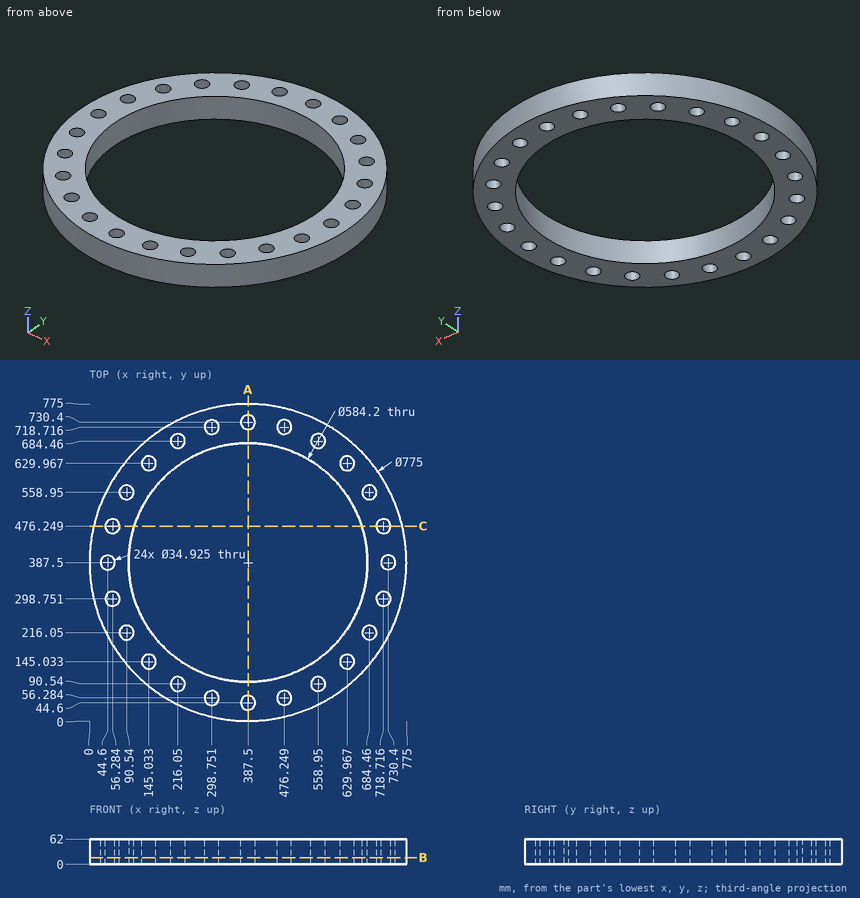
Check sheet for the drawn part. Datum: minimum x, y, z corner. Units: mm. Round coordinates to 2 decimals unless told otherwise and drop trailing zeros. Order: outer loops, then holes, each group sorted by start corner. A loop starts at its lowest first (then second) coordinate and runs counter-clockwise, first axis right, second up. Notation, with made-up numbers: (80.25, -37) -> (93.25, -37) arc R36 cw to (93.25, -3) -> close; hole circle Ø9 at (69, -39.5). An arc over 180 degrees is marked (long way). Use CSV: the item, a comma, the result in double quotes.
(1) Depth check by flat-ended pin: pin 1 (4 mm diameter, centred on y = 257.5, z = 25.5, fed in from -X); pin 2 (12 mm diameter, centred on y = 289.5, z = 34, fed in from +X); pin 3 (3 mm diameter, centred on y = 176.5, z = 12.5, fed in from +X) (1 decimal); pin 4 (21 mm diameter, centred on x = 684.46, y = 558.95, fed in from -Z). Enter the tip coordinate at first touch or a pass-through.
Worked out:
pin 1,"x = 21.75"
pin 2,"x = 763.92"
pin 3,"x = 713.5"
pin 4,"through"
(2) Cross-section at A-A (x = 387.5). Record the boundary of the cut face in (y, z).
Worked out:
outline,"(0, 0) -> (27.14, 0) -> (27.14, 62) -> (0, 62) -> close; (62.06, 0) -> (95.4, 0) -> (95.4, 62) -> (62.06, 62) -> close; (679.6, 0) -> (712.94, 0) -> (712.94, 62) -> (679.6, 62) -> close; (747.86, 0) -> (775, 0) -> (775, 62) -> (747.86, 62) -> close"
(3) Cross-section at C-C (y = 476.5). Record the boundary of the cut face in (x, z).
Worked out:
outline,"(10.36, 0) -> (38.82, 0) -> (38.82, 62) -> (10.36, 62) -> close; (73.74, 0) -> (109.29, 0) -> (109.29, 62) -> (73.74, 62) -> close; (665.71, 0) -> (701.26, 0) -> (701.26, 62) -> (665.71, 62) -> close; (736.18, 0) -> (764.64, 0) -> (764.64, 62) -> (736.18, 62) -> close"
(4) Cross-section at B-B (z = 16.5). Count the separate pieces of the cut face and the enclosed holes in it, and give its area (3 significant figures).
Worked out:
separate pieces,"1"
enclosed holes,"25"
area,"181,000 mm²"
(5) Material ranges on line 1 along X through (y, z) = (387, 15); line 2 along X through (y, z) = (66, 23); line 3 along X through (y, z) = (216, 22), recorded low to high. Write a range as from..to.
Worked out:
line 1,"0..27.14, 62.06..95.4, 679.6..712.94, 747.86..775"
line 2,"171.18..284.24, 313.26..461.74, 490.76..603.82"
line 3,"40.02..73.08, 108..151.05, 623.95..667, 701.92..734.98"
